Verification items for the finished model (mm, model axes). Round coordinates to 2 decimals unless told otherwise and drop trailing zeros. Loops run counter-clockwise (first coordinate to the right, second up) from the corner with the lowest first, then second, coordinate; pieces in that order, holes last.
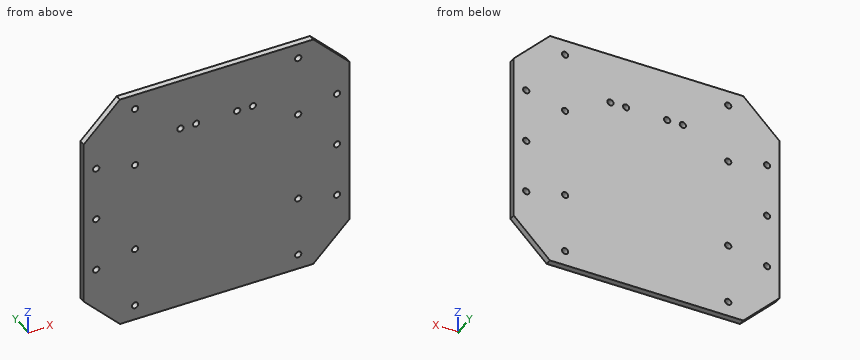
from build123d import *

# Parameters (mm, degrees)
SKETCH2_R           = 3.302
BOSS_EXTRUDE1_DEPTH = 6.35
SKETCH3_R           = 3.302
CUT_EXTRUDE1_DEPTH  = 7.35
SKETCH4_R           = 3.302
CUT_EXTRUDE2_DEPTH  = 7.35


with BuildPart() as part:
    # Sketch2 → Boss-Extrude1 (new body)
    with BuildSketch(Plane(origin=(0, 0, 0), x_dir=(1, 0, 0), z_dir=(0, 1, 0))):
        Polygon((-139.7, -88.9), (-139.7, 88.9), (-101.6, 127), (101.6, 127), (139.7, 88.9), (139.7, -88.9), (101.6, -127), (-101.6, -127), align=None)
        with Locations((-21.59, -73.025)):
            Circle(SKETCH2_R, mode=Mode.SUBTRACT)
        with Locations((-38.1, -73.025)):
            Circle(SKETCH2_R, mode=Mode.SUBTRACT)
        with Locations((38.1, -73.025)):
            Circle(SKETCH2_R, mode=Mode.SUBTRACT)
        with Locations((21.59, -73.025)):
            Circle(SKETCH2_R, mode=Mode.SUBTRACT)
    extrude(amount=BOSS_EXTRUDE1_DEPTH)

    # Sketch3 → Cut-Extrude1 (cut, through all)
    with BuildSketch(Plane(origin=(0, 6.35, 0), x_dir=(1, 0, 0), z_dir=(0, 1, 0))):
        with Locations((-126.619, 57.15)):
            Circle(SKETCH3_R)
        with Locations((-126.619, -57.15)):
            Circle(SKETCH3_R)
        with Locations((126.619, -57.15)):
            Circle(SKETCH3_R)
        with Locations((126.619, 0)):
            Circle(SKETCH3_R)
        with Locations((126.619, 57.15)):
            Circle(SKETCH3_R)
        with Locations((-126.619, 0)):
            Circle(SKETCH3_R)
    extrude(amount=-CUT_EXTRUDE1_DEPTH, mode=Mode.SUBTRACT)

    # Sketch4 → Cut-Extrude2 (cut, through all)
    with BuildSketch(Plane.XZ):
        with Locations((-85.725, 111.125)):
            Circle(SKETCH4_R)
        with Locations((-85.725, -111.125)):
            Circle(SKETCH4_R)
        with Locations((85.725, -111.125)):
            Circle(SKETCH4_R)
        with Locations((85.725, -47.625)):
            Circle(SKETCH4_R)
        with Locations((85.725, 47.625)):
            Circle(SKETCH4_R)
        with Locations((85.725, 111.125)):
            Circle(SKETCH4_R)
        with Locations((-85.725, 47.625)):
            Circle(SKETCH4_R)
        with Locations((-85.725, -47.625)):
            Circle(SKETCH4_R)
    extrude(amount=-CUT_EXTRUDE2_DEPTH, mode=Mode.SUBTRACT)


solid = part.part
1. Section check D-D (z = 97). Enter the section's corners in (x, y).
2. Section check C-C (y = 4). Give the number of separate pieces and of enclosed holes in the cut face, then the cut area to 3 significant figures.
3. Section check A-A (z = -57.15). Enter the section's corners in (x, y).
4. Gauge pin test, flat end, axial feed: P1, Ø5.5, axis at x = 126.619, z = -57.15, coming from the +Y side. Record the tip position at first contact, or that the pin passes through.
5. Scan lines: L1, parallel to X at y = 4.25, z = -57.15; L2, parallel to Z at x = 85.5, y = 3.5; L3, parallel to Z at x = -124.5, y = 1.5. Record each from-to range of solid material in increasing order.
6. Section check B-B (x = -38.1). Enter the section's corners in (y, z).
Taken from the geometry:
1. outline: (-131.6, 0) - (131.6, 0) - (131.6, 6.35) - (-131.6, 6.35) - close
2. separate pieces: 1
2. enclosed holes: 18
2. area: 67,400 mm2
3. outline: (-139.7, 0) - (-129.92, 0) - (-129.92, 6.35) - (-139.7, 6.35) - close; (-123.32, 0) - (123.32, 0) - (123.32, 6.35) - (-123.32, 6.35) - close; (129.92, 0) - (139.7, 0) - (139.7, 6.35) - (129.92, 6.35) - close
4. P1: passes through
5. L1: x = -139.7 to -129.92, -123.32 to 123.32, 129.92 to 139.7
5. L2: z = -127 to -114.42, -107.83 to -50.92, -44.33 to 44.33, 50.92 to 107.83, 114.42 to 127
5. L3: z = -104.1 to -59.68, -54.62 to -2.53, 2.53 to 54.62, 59.68 to 104.1
6. outline: (0, -127) - (6.35, -127) - (6.35, 69.72) - (0, 69.72) - close; (0, 76.33) - (6.35, 76.33) - (6.35, 127) - (0, 127) - close
